Geometry: final body of the model. Coordinates: model frame, mm. A direction names the side the tool comes from. Give positions to 0.01 mm unless a question says otherwise; leave off trailing zeros. Order: outer loops, then holes, each group sorted by start corner. A loop starts at its lowest first (then second) coordinate and runs counter-clockwise, first axis right, second up. Notation, with made-up numbers: (-11, 58.25) - (15, 58.25) arc R15 ccw to (15, 83.25) - close; hole circle Ø9 at (10, 46). An arc over 180 degrees is marked (long way). Put each result on its own line as item: value. Start each with the question number.
1. First-contact query: P1, Ø3, axis at x = 23, z = -81.5, coming from the +Y side; P2, Ø10, axis at x = -26, z = -78, coming from the -Y side. Flat tips, straight axial feed; report the tip coordinate or a pass-through.
2. Section C-C on y = -62.5. Return the cut outline in (x, z).
3. Ray query, line 1 along X through (y, z) = (122.25, -80.5); line 2 along Z through (x, y) = (-25, 120.5); line 3 along Y through (x, z) = (86, -71). Return the intervals inside material, ascending. Write a range as from..to.
4. Section B-B on z = -72.5. Return the cut outline in (x, y), plus the area to 3 significant figures.
5. Mould query, pull axis Y, two halves, no side actions, for faces 4 (the flat face through (2, 125, -80)), 5 (the flat face through (-2, 85, -93)), 6 (the flat face through (85, -25, -73)). Classes: pulls with the +Y half, pulls with the -Y half, needs draft (parallel to the pull), parting line crosses it, or undercut.
6. Section A-A on x = 25. Return the cut outline in (y, z).
7. Set-up query: faces 1 (the flat face through (-95, -25, -73)), 2 (the flat face through (25, 113, -81)), 3 (the flat face through (90, -125, -80)). Return all of +Z, -Z, +X, -X, +Y, -Y with unobstructed straight access to the full face (end or side cutting, diameter ignored); none if empty.
8. Section D-D on y = -104. Return the cut outline in (x, z).
from build123d import *

# Parameters (mm, degrees)
F1_DEPTH = 25
F2_R     = 5
F3_DEPTH = 12
F4_W     = 10
F4_H     = 20
F5_DEPTH = 10


with BuildPart() as f1:
    # F0 (on Top) → F1 (new body)
    with BuildSketch(Plane.XY):
        Polygon((110, -125), (110, 125), (-110, 125), (-110, -125), (-70, -125), (-49.67048, 65.990649), (50.32952, 65.990649), (70, -125), align=None)
    extrude(amount=F1_DEPTH)

    # F2 (on face) → F3 (cut)
    with BuildSketch(Plane(origin=(0, 125, 0), x_dir=(-1, 0, 0), z_dir=(0, 1, 0))):
        with Locations((95, 12.5)):
            Circle(F2_R)
        with Locations((25, 12.5)):
            Circle(F2_R)
        with Locations((-25, 12.5)):
            Circle(F2_R)
        with Locations((-95, 12.5)):
            Circle(F2_R)
    extrude(amount=-F3_DEPTH, mode=Mode.SUBTRACT)

    # F4 (on face) → F5 (cut)
    with BuildSketch(Plane(origin=(0, 0, 0), x_dir=(1, 0, 0), z_dir=(0, 0, -1))):
        with Locations((-90, 25)):
            Rectangle(F4_W, F4_H)
        with Locations((90, 25)):
            Rectangle(F4_W, F4_H)
    extrude(amount=-F5_DEPTH, mode=Mode.SUBTRACT)


with BuildPart() as f7_1:
    # F7: instance of F1
    add(f1.part.mirror(Plane.XY.offset(-34)))


solid = f7_1.part
Resolved:
1. P1: y = 113
1. P2: y = 65.99
2. outline: (-110, -93) - (-63.35, -93) - (-63.35, -68) - (-110, -68) - close; (63.56, -93) - (110, -93) - (110, -68) - (63.56, -68) - close
3. line 1: -110..-100, -90..-30, -20..20, 30..90, 100..110
3. line 2: -93..-85.5, -75.5..-68
3. line 3: -125..-35, -15..125
4. outline: (-110, -125) - (-70, -125) - (-49.67, 65.99) - (50.33, 65.99) - (70, -125) - (110, -125) - (110, 125) - (-110, 125) - close; hole (-95, -35) - (-85, -35) - (-85, -15) - (-95, -15) - close; hole (85, -35) - (95, -35) - (95, -15) - (85, -15) - close
4. area: 31,700 mm^2
5. face 4: pulls with the +Y half
5. face 5: needs draft
5. face 6: undercut
6. outline: (65.99, -93) - (125, -93) - (125, -85.5) - (113, -85.5) - (113, -75.5) - (125, -75.5) - (125, -68) - (65.99, -68) - close
7. face 1: +Z
7. face 2: +Y
7. face 3: +Z, -Z, +X, -X, -Y
8. outline: (-110, -93) - (-67.76, -93) - (-67.76, -68) - (-110, -68) - close; (67.84, -93) - (110, -93) - (110, -68) - (67.84, -68) - close
